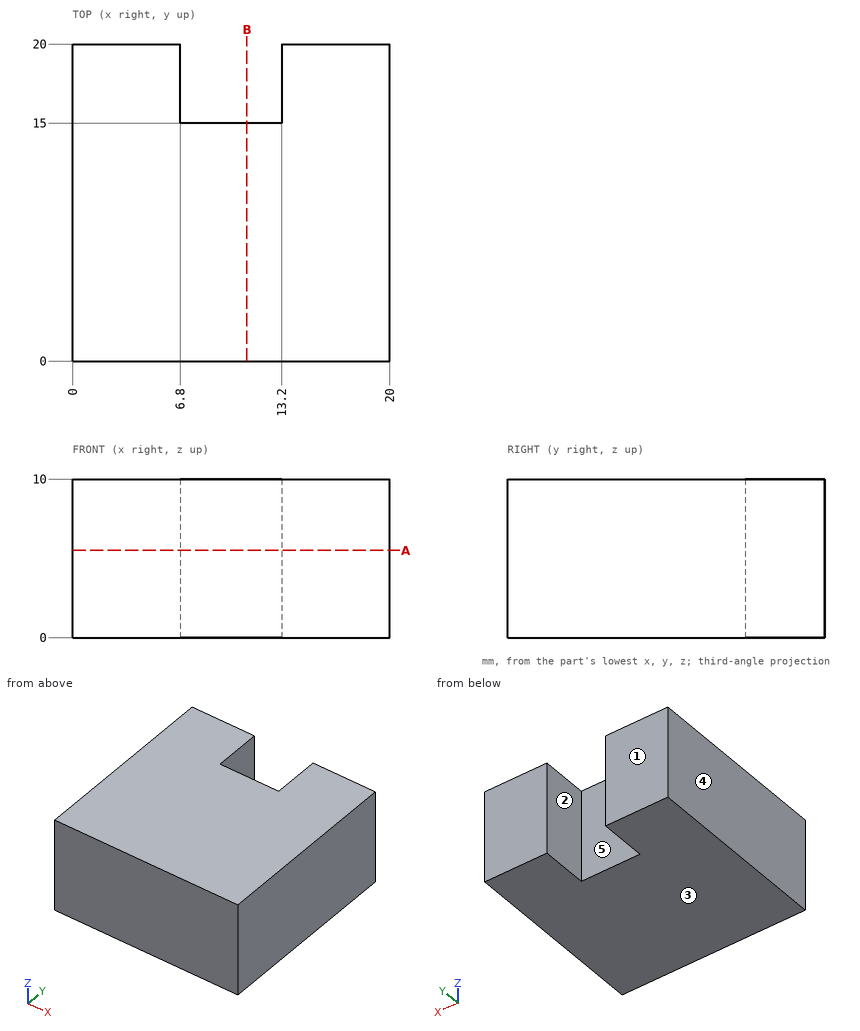
Geometry check sheet. Reference: drawing and pictorial views, mm from the part's lowest x, y, z. A direction names the side the tool comes from. Coordinates: 2 decimals unless noted, no trailing zeros. Order: outer loops, then holes, each group sorted by start corner. A loop starts at its lowest first (then second) coordinate and runs counter-clockwise, first axis right, second up.
Item 1: Release check for a two-part mould opening along X. For the marked faces 3, 4 and 5 record: +X half, -X half, draft (parallel to the pull), parting line (faces both ways), or undercut.
Filled in:
face 3: draft
face 4: -X half
face 5: undercut
Item 2: Section check A-A, the plane z = 5.5. Enter the section's corners in (x, y), then the cut area to 3 significant figures.
Filled in:
outline: (0, 0) - (20, 0) - (20, 20) - (13.2, 20) - (13.2, 15) - (6.8, 15) - (6.8, 20) - (0, 20) - close
area: 368 mm2
Item 3: Access from +Z, -Z, +X, -X, +Y, -Y to the whole of each face (thin tool, end or side, straight path). Record for the marked faces 1 and 2.
Filled in:
face 1: +Z, -Z, +X, -X, +Y
face 2: +Z, -Z, +Y
Item 4: Section check B-B, the plane x = 11. Enter the section's corners in (y, z), then the cut area to 3 significant figures.
Filled in:
outline: (0, 0) - (15, 0) - (15, 10) - (0, 10) - close
area: 150 mm2
Item 5: Material ranges on L1, parallel to X at y = 17, z = 9; L2, parallel to Y at x = 7.5, z = 8.5, recorded low to high.
Filled in:
L1: x = 0 to 6.8, 13.2 to 20
L2: y = 0 to 15
Item 6: Depth check by flat-ended pin: pin 1 (5 mm diameter, centred on x = 10, z = 4.5, fed in from +Y); pin 2 (4 mm diameter, centred on x = 4.5, z = 6, fed in from -Y). Enter the tip coordinate at first touch or a pass-through.
Filled in:
pin 1: stops at y = 15
pin 2: stops at y = 0
